```python
from build123d import *

# Parameters (mm, degrees)
SKETCH1_R           = 28
BOSS_EXTRUDE1_DEPTH = 41
SKETCH2_R           = 10.05
CUT_EXTRUDE1_DEPTH  = 8.1
SKETCH3_R           = 4.05
CUT_EXTRUDE2_DEPTH  = 64.757352517


with BuildPart() as part:
    # Sketch1 → Boss-Extrude1 (new body)
    with BuildSketch(Plane(origin=(0, 0, 0), x_dir=(0, 0, -1), z_dir=(1, 0, 0))):
        Circle(SKETCH1_R)
        with BuildLine():
            Line((-15.609520213, 40), (-12.609520213, 25))
            ThreePointArc((-12.609520213, 25), (0, 28), (12.609520213, 25))
            Line((12.609520213, 25), (15.609520213, 40))
            Line((15.609520213, 40), (-15.609520213, 40))
        make_face()
    extrude(amount=BOSS_EXTRUDE1_DEPTH)

    # Sketch2 → Cut-Extrude1 (cut)
    with BuildSketch(Plane(origin=(0, 0, 0), x_dir=(0, 0, -1), z_dir=(1, 0, 0))):
        Circle(SKETCH2_R)
    extrude(amount=CUT_EXTRUDE1_DEPTH, mode=Mode.SUBTRACT)

    # Sketch3 → Cut-Extrude2 (cut, through all)
    with BuildSketch(Plane(origin=(0, 0, 0), x_dir=(0, 0, -1), z_dir=(1, 0, 0))):
        Circle(SKETCH3_R)
    extrude(amount=CUT_EXTRUDE2_DEPTH, mode=Mode.SUBTRACT)


solid = part.part
```
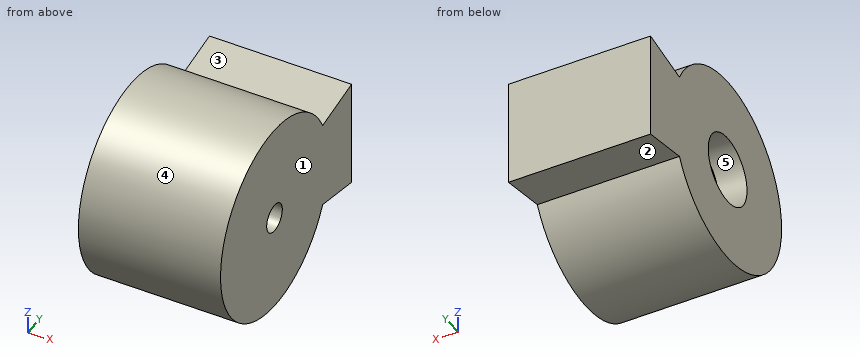
Here's how the part is built. I have some questions about the finished solid (model axes, mm). Face numbers are marked on the shaded views. A direction names the side the tool comes from. Give positions to 0.01 mm unless a question says otherwise; leave off trailing zeros. Write each loop counter-clockwise with the first axis right and the second up, starting at its lowest first coordinate (ties: lowest second). Pieces come first, ordered by that corner, then holes. Notation, with made-up numbers: (-24.5, 26) -> (-7.5, 26) arc R27 cw to (-7.5, 42) -> close; hole circle Ø6 at (17, 24). An arc over 180 degrees is marked (long way). Write each question's results on one line, items separated by ' | '.
Item 1: Suppose I cut it at A-A on z = 0. Write out the boundary of the cut face in (x, y).
Output:
outline: (0, -28) -> (41, -28) -> (41, -4.05) -> (8.1, -4.05) -> (8.1, -10.05) -> (0, -10.05) -> close; (0, 10.05) -> (8.1, 10.05) -> (8.1, 4.05) -> (41, 4.05) -> (41, 40) -> (0, 40) -> close
Item 2: Suppose I cut it at C-C on x = 13. Write out the boundary of the cut face in (y, z).
Output:
outline: (25, -12.61) -> (40, -15.61) -> (40, 15.61) -> (25, 12.61) arc R28 ccw (long way) to start; hole circle Ø8.1 at (0, 0)
Item 3: Suppose I cut it at B-B on y = 0. Write out the boundary of the cut face in (x, z), plus the area to 3 significant figures.
Output:
outline: (0, -28) -> (41, -28) -> (41, -4.05) -> (8.1, -4.05) -> (8.1, -10.05) -> (0, -10.05) -> close; (0, 10.05) -> (8.1, 10.05) -> (8.1, 4.05) -> (41, 4.05) -> (41, 28) -> (0, 28) -> close | area: 1,870 mm^2
Item 4: On a 3-axis mill with a long thin cutter (end or side, diameter ignored), from which of +Z, -Z, +X, -X, +Y, -Y can I reach the whole of each face in a straight line? I mean the marked faces 1 and 2. Say none if no direction works.
Output:
face 1: +Z, -Z, +X, +Y, -Y | face 2: -Z, +X, -X
Item 5: We'd pull the mould along Z, two halves only. Please class the marked faces 3, 4 and 5: pulls with the +Z half, pulls with the -Z half, needs draft (parallel to the pull), parting line crosses it, or undercut.
Output:
face 3: pulls with the +Z half | face 4: parting line crosses it | face 5: undercut
Item 6: Suppose I cut it at D-D on y = 7. Write out the boundary of the cut face in (x, z).
Output:
outline: (0, -27.11) -> (41, -27.11) -> (41, 27.11) -> (0, 27.11) -> (0, 7.21) -> (8.1, 7.21) -> (8.1, -7.21) -> (0, -7.21) -> close
Item 7: For pin 1 Ø6 at (x, z) = (20, -22.5) entering from -Y; pin 2 Ø12 at (x, z) = (32, -11.5) entering from -Y; pin 3 Ø13 at (y, z) = (0, 0) entering from +X; pin 4 Ø8 at (x, y) = (25, 17) entering from -Z, each with a flat end and sliding along its axis, tell me the tip position at first contact or that it passes through.
Output:
pin 1: stops at y = -20.09 | pin 2: stops at y = -27.45 | pin 3: stops at x = 41 | pin 4: stops at z = -24.8
Item 8: If I drill on L1, parallel to Y at x = 20, z = 0; L2, parallel to Z at x = 27, y = 0; L3, parallel to Y at x = 3, z = 0, over which ranges is the centre line in solid material (lowest first)?
Output:
L1: y = -28 to -4.05, 4.05 to 40 | L2: z = -28 to -4.05, 4.05 to 28 | L3: y = -28 to -10.05, 10.05 to 40
